```python
from build123d import *

# Parameters (mm, degrees)
F0_R     = 1.05
F1_DEPTH = 1.5


with BuildPart() as f1:
    # F0 (on Front) → F1 (new body)
    with BuildSketch(Plane.XZ):
        Polygon((13.033743, -10.610216), (13.033743, 18.713196), (-16.966257, 18.713196), (-16.966257, -14.286804), (9.357155, -14.286804), align=None)
        with Locations((-15.025558, -12.278115)):
            Circle(F0_R, mode=Mode.SUBTRACT)
        with Locations((11.168605, 16.665677)):
            Circle(F0_R, mode=Mode.SUBTRACT)
    extrude(amount=-F1_DEPTH)


solid = f1.part
```
Here's how the part is built. I have some questions about the finished solid (model axes, mm). Coordinates: 2 decimals unless noted, no trailing zeros. Loops run counter-clockwise (first coordinate to the right, second up) from the corner with the lowest first, then second, coordinate; pieces in that order, holes last. Notation, with made-up numbers: (-15.75, 89.5) -> (-10.75, 89.5) arc R16 ccw to (-10.75, 93.5) -> close; hole circle Ø6 at (-39, 67.25). An arc over 180 degrees is marked (long way). Return JSON: item names as keys, results as strings.
1) Thinking about a two-plate mould opening in Z: for faces 1 (the face through (-16.966, 1, 2)), 2 (the face through (11.17, 0.74, -12.474)), 3 (the face through (-14.461, 0.74, -11.393)), 4 (the face through (-2, 1, 18.713)), which applies, +Z half, -Z half, draft (parallel to the pull), parting line (faces both ways), or undercut?
Results below:
{"face 1": "draft", "face 2": "-Z half", "face 3": "undercut", "face 4": "+Z half"}
2) If we section it at A-A, the plane x = 11: Write out the boundary of the cut face in (y, z), then the cut area to 3 significant figures.
Results below:
{"outline": "(0, -12.64) -> (1.5, -12.64) -> (1.5, 15.63) -> (0, 15.63) -> close; (0, 17.7) -> (1.5, 17.7) -> (1.5, 18.71) -> (0, 18.71) -> close", "area": "43.9 mm²"}
3) I need wall thicknesses on line 1 (Z direction, x = 10.25, y = 1.3); line 2 (X direction, y = 0.1, z = 16.5); line 3 (X direction, y = 0.5, z = -13). Which ranges of each line are inside material? Lowest first, please. Write a range as from..to.
Results below:
{"line 1": "-13.39..16.16, 17.17..18.71", "line 2": "-16.97..10.13, 12.21..13.03", "line 3": "-16.97..-15.79, -14.26..10.64"}
